Source: CAD feature listing. Evaluate the final solid. Frame: model axes, mm. A direction names the side the tool comes from. Give positions to 0.01 mm unless a question says otherwise; leave off trailing zeros. Order: outer loops, then holes, each group sorted by start corner. A loop starts at its lowest first (then second) coordinate and runs counter-clockwise, first axis right, second up. Notation, with made-up numbers: M 21.25,-37.75 L 67.25,-37.75 A13 ccw 67.25,-15.75 Z; hole C 10,-1.75 d3. An arc over 180 degrees is marked long. Answer as a JSON object with one key per item and string values. Group by question number.
1. Section query C-C (y = 45.5). Count the separate pieces of the cut face and the enclosed holes in it, plus the area to 3 significant figures.
2. Material intervals for L1, parallel to Y at x = 0, z = 13.15; L2, parallel to Y at x = 0, z = 11.25; L3, parallel to Z at x = 0, y = 48, sorted ascending. Write a range as [from, to].
3. Section query D-D (z = 4.25). Output: boundary loops of the cut face in (x, y), plus the area to 3 significant figures.
4. Pin query (flat end, axial travel): P1, Ø1.8, axis at y = 44, z = 7, coming from the +X side; P2, Ø7, axis at x = -2, y = 48.5, coming from the +Z side; P3, Ø4, axis at x = 14, z = 10.5, coming from the +Y side; P4, Ø6.5, axis at x = 3, z = 3.5, coming from the -Y side. Return the tip coordinate at first contact, or that it passes through.
5. Set-up query: faces 1 (the flat face through (41, -37, 14)), 2 (the cylindrical face through (-0.867, 48.658, 2.595)), 3 (the flat face through (0, 42, 2)), 4 (the flat face through (0, 47, 13)). Return all of +Z, -Z, +X, -X, +Y, -Y with unobstructed straight access to the full face (end or side cutting, diameter ignored); none if empty.
6. Pull-direction query (X, two-part tool) for faces 5 (the flat face through (38.1, -34.3, 14)), 6 (the cylindrical face through (-11.056, -49.787, 6.902)), 7 (the cylindrical face through (52.937, 16.671, 6.902)), 8 (the flat face through (-10, 48, 7)); classes: +X half, -X half, draft (parallel to the pull), parting line (faces both ways), or undercut.
7. Section query A-A (x = 0). Output: boundary loops of the cut face in (y, z).
8. Section query B-B (y = 0). Output: boundary loops of the cut face in (x, z).
from build123d import *

# Parameters (mm, degrees)
SKETCH_R        = 55.5
SKETCH_R_2      = 51
PAD_DEPTH       = 14
SKETCH001_R     = 54
SKETCH001_R_2   = 52.5
POCKET_DEPTH    = 1
SKETCH003_W     = 15
SKETCH003_H     = 13
PAD001_DEPTH    = 10
SKETCH004_W     = 24
SKETCH004_H     = 13
PAD002_DEPTH    = 4
SKETCH002_R     = 4
POCKET001_DEPTH = 55.501
CHAMFER_SIZE    = 0.7
CHAMFER001_SIZE = 0.7


with BuildPart() as part:
    # Sketch → Pad (new body)
    with BuildSketch(Plane.XY):
        Circle(SKETCH_R)
        Circle(SKETCH_R_2, mode=Mode.SUBTRACT)
    extrude(amount=PAD_DEPTH)

    # Sketch001 (on Face4 of Pad) → Pocket (cut)
    with BuildSketch(Plane.XY.offset(14)):
        Circle(SKETCH001_R)
        Circle(SKETCH001_R_2, mode=Mode.SUBTRACT)
    extrude(amount=-POCKET_DEPTH, mode=Mode.SUBTRACT)

    # Sketch003 → Pad001 (join)
    with BuildSketch(Plane.XZ.offset(-52)):
        with Locations((0, 6.5)):
            Rectangle(SKETCH003_W, SKETCH003_H)
    extrude(amount=PAD001_DEPTH)

    # Sketch004 → Pad002 (join)
    with BuildSketch(Plane.XZ.offset(-52)):
        with Locations((0, 6.5)):
            Rectangle(SKETCH004_W, SKETCH004_H)
    extrude(amount=PAD002_DEPTH)

    # Sketch002 → Pocket001 (cut, through all)
    with BuildSketch(Plane.XZ):
        with Locations((0, 6.5)):
            Circle(SKETCH002_R)
    extrude(amount=-POCKET001_DEPTH, mode=Mode.SUBTRACT)

    # Chamfer
    chamfer_edges = [part.edges().sort_by_distance(p)[0] for p in [
        (-52.5, 0, 14),
    ]]
    chamfer(chamfer_edges, length=CHAMFER_SIZE)

    # Chamfer001
    chamfer001_edges = [part.edges().sort_by_distance(p)[0] for p in [
        (-54, 0, 14),
    ]]
    chamfer(chamfer001_edges, length=CHAMFER001_SIZE)


solid = part.part
Answer sheet:
{
 "1": {"separate pieces": "3", "enclosed holes": "1", "area": "382 mm^2"},
 "2": {"L1": "[-55.5, -54], [-52.5, -51], [51, 52.5], [54, 55.5]", "L2": "[-55.5, -51], [42, 55.5]", "L3": "[0, 2.5], [10.5, 13]"},
 "3": {"outline": "M -12,48 L -7.5,48 L -7.5,42 L -3.31,42 L -3.31,55.4 A55.5 ccw long 3.31,55.4 L 3.31,42 L 7.5,42 L 7.5,48 L 12,48 L 12,49.57 A51 cw long -12,49.57 Z", "area": "1,570 mm^2"},
 "4": {"P1": "x = 34.97", "P2": "z = 14", "P3": "y = 54.19", "P4": "y = -55.5"},
 "5": {"face 1": "+Z, +X, -X, +Y, -Y", "face 2": "+Y", "face 3": "+Z, -Z", "face 4": "+Z"},
 "6": {"face 5": "draft", "face 6": "undercut", "face 7": "parting line", "face 8": "undercut"},
 "7": {"outline": "M -55.5,0 L -51,0 L -51,14 L -51.8,14 L -52.5,13.3 L -52.5,13 L -54,13 L -54,13.3 L -54.7,14 L -55.5,14 Z; M 42,0 L 55.5,0 L 55.5,2.5 L 42,2.5 Z; M 42,10.5 L 55.5,10.5 L 55.5,14 L 54.7,14 L 54,13.3 L 54,13 L 52.5,13 L 52.5,13.3 L 51.8,14 L 51,14 L 51,13 L 42,13 Z"},
 "8": {"outline": "M -55.5,0 L -51,0 L -51,14 L -51.8,14 L -52.5,13.3 L -52.5,13 L -54,13 L -54,13.3 L -54.7,14 L -55.5,14 Z; M 51,0 L 55.5,0 L 55.5,14 L 54.7,14 L 54,13.3 L 54,13 L 52.5,13 L 52.5,13.3 L 51.8,14 L 51,14 Z"}
}
